from build123d import *

# Parameters (mm, degrees)
BOSS_EXTRUDE1_DEPTH = 127
CHAMFER1_SIZE       = 0.254


with BuildPart() as part:
    # Sketch1 → Boss-Extrude1 (new body)
    with BuildSketch(Plane.XY):
        with BuildLine():
            Line((2.38125, 5.55625), (-2.38125, 5.55625))
            Line((-2.38125, 5.55625), (-2.38125, 7.571892411))
            ThreePointArc((-2.38125, 7.571892411), (-4.695888328, -6.399417088), (7.9375, 0))
            ThreePointArc((7.9375, 0), (6.399417088, 4.695888328), (2.38125, 7.571892411))
            Line((2.38125, 7.571892411), (2.38125, 5.55625))
        make_face()
    extrude(amount=BOSS_EXTRUDE1_DEPTH)

    # Chamfer1
    chamfer1_edges = [part.edges().sort_by_distance(p)[0] for p in [
        (0, -7.9375, 0),
        (0, -7.9375, 127),
    ]]
    chamfer(chamfer1_edges, length=CHAMFER1_SIZE)


solid = part.part
Could you check a few things on this model? Use its own coordinates, in mm. A direction names the side the tool comes from. Round coordinates to 2 decimals unless told otherwise and drop trailing zeros. Order: outer loops, then holes, each group sorted by start corner. A loop starts at its lowest first (then second) coordinate and runs counter-clockwise, first axis right, second up. Notation, with made-up numbers: M -14.5,-23.5 L 32.5,-23.5 A25 cw 32.5,-1.5 Z; hole C 83,47.25 d1. An arc over 180 degrees is marked long. One line per item, written item: value.
(1) If we mould it in two halves opening along X, with no side actions, what happens to faces 3 (the flat face through (0, 5.556, 63)), 4 (the flat face through (0, 0, 0))? For each: released by +X, released by -X, zero draft, split by the parting line, or undercut.
Ans:
face 3: undercut
face 4: zero draft
(2) Which directions (+Z, -Z, +X, -X, +Y, -Y) give clear straight access to the entire face, cutting with the end or side of a thin tool? Please do faces 1 (the flat face through (2.381, 7, 63)), 2 (the flat face through (0, 0, 127)).
Ans:
face 1: +Z, -Z, +Y
face 2: +Z, +X, -X, +Y, -Y
(3) Imagine slicing it at B-B (x = 0). Write out the boundary of the cut face in (y, z).
Ans:
outline: M -7.94,0.25 L -7.68,0 L 5.56,0 L 5.56,127 L -7.68,127 L -7.94,126.75 Z
(4) I'm going to push flat-ended pins straight in: P1, Ø8, axis at y = 4.5, z = 65.5, coming from the +X side; P2, Ø2.5, axis at x = 1, z = 36, coming from the +Y side; P3, Ø1.6, axis at y = 6, z = 91, coming from the +X side. Where does each tip first touch, or does it pass through?
Ans:
P1: stops at x = 7.92
P2: stops at y = 5.56
P3: stops at x = 6
(5) Imagine slicing it at A-A (z = 62). Write out the boundary of the cut face in (x, y) (1 decimal), and give its area (3 significant figures).
Ans:
outline: M -2.4,5.6 L -2.4,7.6 A7.9 ccw long 2.4,7.6 L 2.4,5.6 Z
area: 187 mm^2
(6) I need wall thicknesses on line 1 along Y through (x, z) = (-0.5, 43); line 2 along X through (y, z) = (2, 88.5); line 3 along Y through (x, z) = (-2, 25.5). Which ranges of each line are inside material? Lowest first, please. Write a range as from..to.
Ans:
line 1: y = -7.92..5.56
line 2: x = -7.68..7.68
line 3: y = -7.68..5.56
